CAD build for the part. Positions are in the model's coordinates, mm. Round coordinates to 2 decimals unless told otherwise and drop trailing zeros.
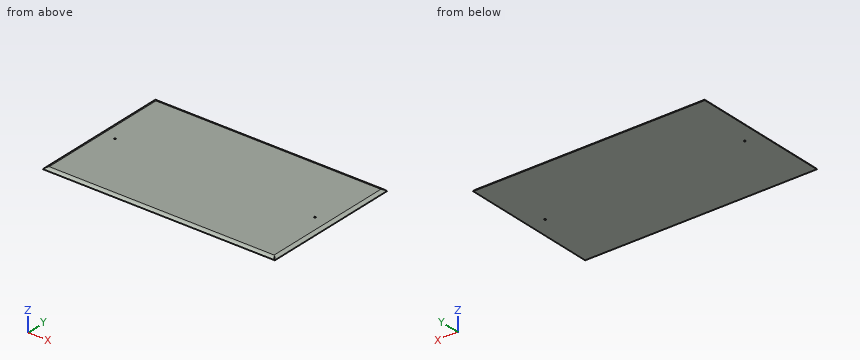
```python
from build123d import *

# Parameters (mm, degrees)
F0_W        = 1416.05
F0_H        = 838.2
F0_R        = 4.7625
F1_DEPTH    = 12.7
F2_T1_DEPTH = 1576.8352262806
F2_T3_DEPTH = 998.9852262806


# Not quite as in the source:
# - a fillet or chamfer that OpenCascade refuses, or shapes differently, is made with other operations: its cross-section is extruded or revolved along the edge and cut away or added
# - a feature names something its author has since deleted; it is built from what else it names


with BuildPart() as f1:
    # F0 (on Top) → F1 (new body)
    with BuildSketch(Plane.XY):
        Polygon((-101.6, 812.8255558279), (-101.6, -76.1744441721), (1365.25, -76.1744441721), (1365.25, 736.6255558279), (1365.25, 812.8255558279), align=None)
        with Locations((631.825, 368.3255558279)):
            Rectangle(F0_W, F0_H, mode=Mode.SUBTRACT)
        with Locations((631.825, 368.3255558279)):
            Rectangle(F0_W, F0_H)
        with Locations((0, 368.3255558279)):
            Circle(F0_R, mode=Mode.SUBTRACT)
        with Locations((1263.65, 368.3255558279)):
            Circle(F0_R, mode=Mode.SUBTRACT)
    extrude(amount=F1_DEPTH)

    # F2: fillet of radius 25.4 on 4 edges, made by hand

    # F2_s2 → F2_t1 (cut)
    with BuildSketch(Plane.YZ.offset(-156.5926131403)):
        with BuildLine():
            ThreePointArc((-76.1744441721, 0), (-66.8773989159, 9.2970452561), (-54.1773989159, 12.7))
            Line((-54.1773989159, 12.7), (-76.1744441721, 12.7))
            Line((-76.1744441721, 12.7), (-76.1744441721, 0))
        make_face()
        with BuildLine():
            ThreePointArc((812.8255558279, 0), (803.5285105718, 9.2970452561), (790.8285105718, 12.7))
            Line((790.8285105718, 12.7), (812.8255558279, 12.7))
            Line((812.8255558279, 12.7), (812.8255558279, 0))
        make_face()
    extrude(amount=F2_T1_DEPTH, mode=Mode.SUBTRACT)

    # F2_s4 → F2_t3 (cut)
    with BuildSketch(Plane.XZ.offset(-867.8181689683)):
        with BuildLine():
            ThreePointArc((-101.6, 0), (-92.3029547439, 9.2970452561), (-79.6029547439, 12.7))
            Line((-79.6029547439, 12.7), (-101.6, 12.7))
            Line((-101.6, 12.7), (-101.6, 0))
        make_face()
        with BuildLine():
            ThreePointArc((1365.25, 0), (1355.9529547439, 9.2970452561), (1343.2529547439, 12.7))
            Line((1343.2529547439, 12.7), (1365.25, 12.7))
            Line((1365.25, 12.7), (1365.25, 0))
        make_face()
    extrude(amount=F2_T3_DEPTH, mode=Mode.SUBTRACT)


solid = f1.part
```
Item 1: Probe line 1 (Y direction, x = 0, z = 9.5); line 2 (Y direction, x = 1263.65, z = 4); line 3 (Y direction, x = 57, z = 2.5). List the from-to ranges inside material, lowest first.
Answers follow:
line 1: y = -66.52 to 363.56, 373.09 to 803.17
line 2: y = -73.32 to 363.56, 373.09 to 809.97
line 3: y = -74.53 to 811.18
Item 2: Flat gauge pins, fed straight in: P1, Ø10, axis at x = 437.5, y = 118, coming from the -Z side; P2, Ø4, axis at y = 609.5, z = 5.5, coming from the -X side; P3, Ø4, axis at y = 302.5, z = 7.5, coming from the +X side; P4, Ø3, axis at x = 496, z = 5.5, coming from the +Y side. Where does each tip first touch, or does it go through?
Answers follow:
P1: stops at z = 0
P2: stops at x = -99.17
P3: stops at x = 1360.97
P4: stops at y = 809.97
Item 3: Cut at A-A, the plane z = 8.5. State how many separate pieces and enclosed holes the cut face has, plus the area to 3 significant figures.
Answers follow:
separate pieces: 1
enclosed holes: 2
area: 1,270,000 mm2
